Here's the drawing with two shaded views (mm, measured from the low corner). I have some questions. Coordinates: 2 decimals unless noted, no trailing zeros. Order: outer loops, then holes, each group sorted by start corner. A loop starts at its lowest first (then second) coordinate and runs counter-clockwise, first axis right, second up. Notation, with made-up numbers: (-1, 12.25) -> (3, 12.25) arc R37 cw to (3, 48.25) -> close; hole circle Ø11 at (34.5, -22.75). An arc over 180 degrees is marked (long way). Write item = value, one per line.
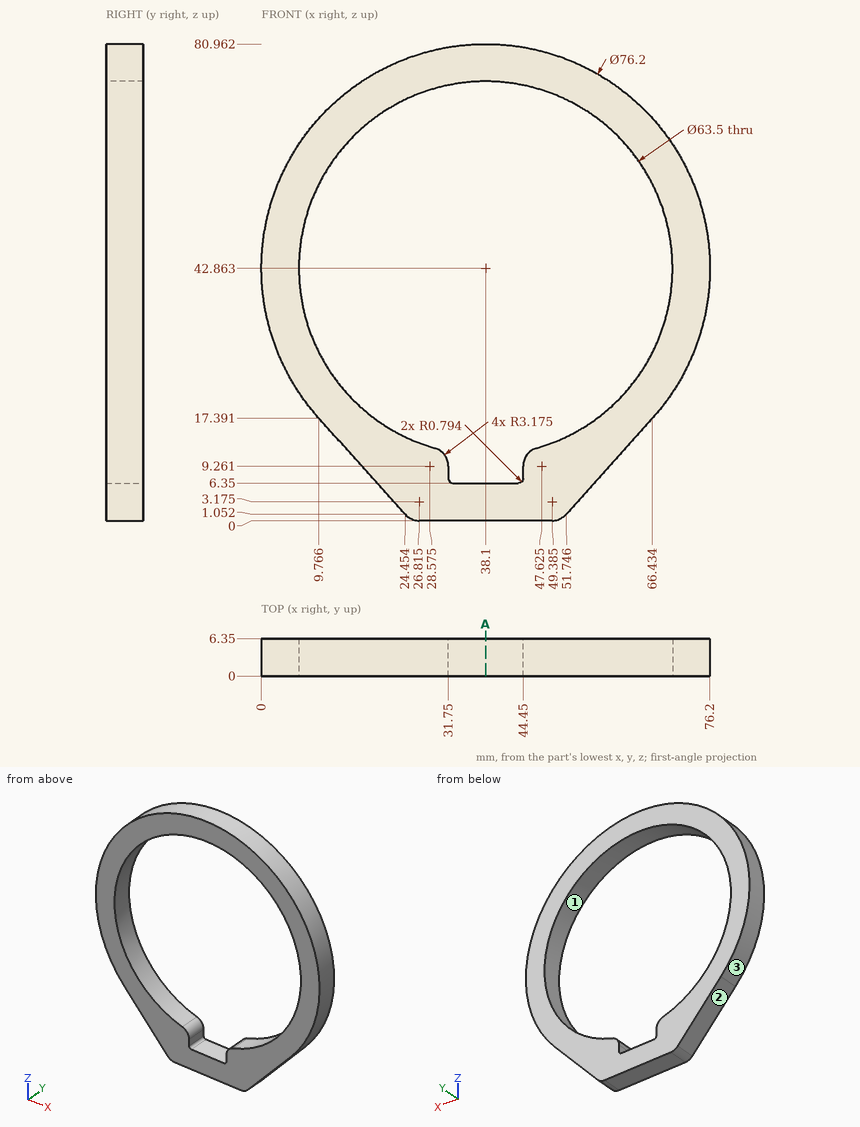
Item 1: I want a section at A-A, the plane x = 38.1. Please give me the cut outline in (y, z).
A:
outline = (0, 0) -> (6.35, 0) -> (6.35, 6.35) -> (0, 6.35) -> close; (0, 74.61) -> (6.35, 74.61) -> (6.35, 80.96) -> (0, 80.96) -> close
Item 2: If we mould it in two halves opening along X, with no side actions, what happens to the marked faces 1, 2 and 3? For each: pulls with the +X half, pulls with the -X half, needs draft (parallel to the pull), parting line crosses it, or undercut.
A:
face_1 = undercut
face_2 = pulls with the -X half
face_3 = parting line crosses it
Item 3: I'm going to push flat-ended pins straight in: P1, Ø0.6, axis at y = 4.5, z = 8, coming from the -X side; P2, Ø1.5, axis at y = 3.5, z = 31, coming from the +X side; P3, Ø1.5, axis at y = 5, z = 12.5, coming from the -X side. Where does each tip first touch, or does it pass through?
A:
P1 = 17.94
P2 = 74.54
P3 = 13.49
Item 4: If I drill on probe 1 along Z at (x, y) = (38.1, 2.25); probe 2 along Z at (x, y) = (39, 2.5); probe 3 along X at (y, z) = (1.25, 22.5), over which ranges is the centre line in solid material (lowest first)?
A:
probe_1 = 0 to 6.35, 74.61 to 80.96
probe_2 = 0 to 6.35, 74.6 to 80.95
probe_3 = 5.9 to 13.74, 62.46 to 70.3
